For this review, take the finished solid that the model builds, in its own axes (mm). Face numbers are marked on the shaded views. A direction names the side the tool comes from. Give positions to 0.01 mm unless a question says otherwise; leave off trailing zeros. Order: outer loops, then holes, each group sorted by start corner. A loop starts at its lowest first (then second) coordinate and runs counter-clockwise, first axis right, second up. Notation, with made-up numbers: (-36, 11.25) - (10, 11.25) arc R18 cw to (10, 45.25) - close; hole circle Ø2 at (-17.75, 6). An arc over 180 degrees is marked (long way). One line per item, written item: value.
```python
from build123d import *

# Parameters (mm, degrees)
SKETCH1_W           = 45
SKETCH1_H           = 19
BOSS_EXTRUDE1_DEPTH = 26
SKETCH2_W           = 48
SKETCH2_H           = 29
BOSS_EXTRUDE2_DEPTH = 2
SKETCH3_W           = 2.4
SKETCH3_H           = 1.6
CUT_EXTRUDE1_DEPTH  = 2


with BuildPart() as part:
    # Sketch1 → Boss-Extrude1 (new body)
    with BuildSketch(Plane(origin=(0, 0, 0), x_dir=(1, 0, 0), z_dir=(0, 1, 0))):
        Rectangle(SKETCH1_W, SKETCH1_H)
    extrude(amount=BOSS_EXTRUDE1_DEPTH)

    # Sketch2 → Boss-Extrude2 (add)
    with BuildSketch(Plane.XY.offset(9.5)):
        with Locations((0, 13)):
            Rectangle(SKETCH2_W, SKETCH2_H)
    extrude(amount=BOSS_EXTRUDE2_DEPTH)

    # Sketch3 → Cut-Extrude1 (cut)
    with BuildSketch(Plane(origin=(0, 26, 0), x_dir=(1, 0, 0), z_dir=(0, 1, 0))):
        with Locations((-0.003209451, -7.489007977)):
            Rectangle(SKETCH3_W, SKETCH3_H)
    extrude(amount=-CUT_EXTRUDE1_DEPTH, mode=Mode.SUBTRACT)


solid = part.part
```
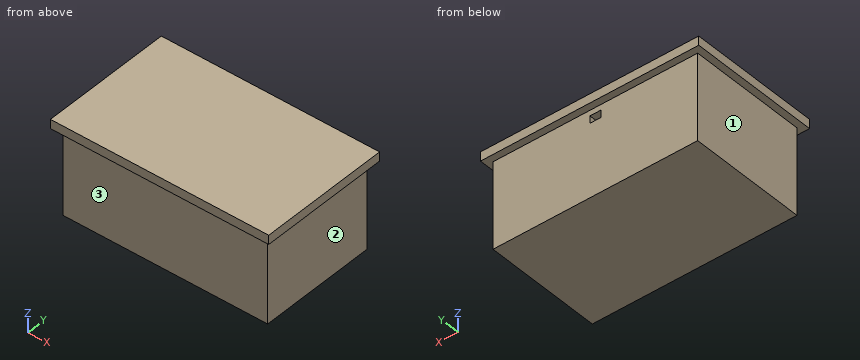
(1) Take a section at C-C (z = 4.25). Write out the cut boundary in (x, y), then the cut area to 3 significant figures.
Answers below:
outline: (-22.5, 0) - (22.5, 0) - (22.5, 26) - (-22.5, 26) - close
area: 1,170 mm^2
(2) Take a section at B-B (x = -7.5). Write out the cut boundary in (y, z).
Answers below:
outline: (-1.5, 9.5) - (0, 9.5) - (0, -9.5) - (26, -9.5) - (26, 9.5) - (27.5, 9.5) - (27.5, 11.5) - (-1.5, 11.5) - close
(3) For P1, Ø8, axis at x = 8, z = 8.5, coming from the +Y side; P2, Ø0.8, axis at x = 0, z = 7.5, coming from the +Y side; P3, Ø1.8, axis at y = 25, z = 7.5, coming from the +X side; P4, Ø2, axis at y = 2, z = -2, coming from the -X side, all flat-tipped, find the tip position at first contact; note any pin that passes through.
Answers below:
P1: stops at y = 27.5
P2: stops at y = 24
P3: stops at x = 22.5
P4: stops at x = -22.5
(4) Wall thickness on line 1 (Y direction, x = -6.5, z = -2.75); line 2 (X direction, y = 2.75, z = 5.75): over which ranges is each line inside the solid? List them lowest first. Write a range as from..to.
Answers below:
line 1: y = 0..26
line 2: x = -22.5..22.5
(5) Machinability: for the marked faces 1, 2 and 3, which of the approach directions +Z, -Z, +X, -X, +Y, -Y give a long, thin tool a straight path to every point of the face, cutting with its end or side? Answer none if there is none.
Answers below:
face 1: -Z, -X, +Y, -Y
face 2: -Z, +X, +Y, -Y
face 3: -Z, +X, -X, -Y
(6) Take a section at A-A (y = 12). Write out the cut boundary in (x, z), then the cut area to 3 significant figures.
Answers below:
outline: (-24, 9.5) - (-22.5, 9.5) - (-22.5, -9.5) - (22.5, -9.5) - (22.5, 9.5) - (24, 9.5) - (24, 11.5) - (-24, 11.5) - close
area: 951 mm^2
